from build123d import *

# Parameters (mm, degrees)
BOSS_EXTRUDE1_DEPTH = 20
SKETCH2_R           = 3.15
CUT_EXTRUDE2_DEPTH  = 11
SKETCH3_R           = 4.25
CUT_EXTRUDE3_DEPTH  = 4
BOSS_EXTRUDE2_DEPTH = 5


with BuildPart() as part:
    # Sketch1 → Boss-Extrude1 (new body)
    with BuildSketch(Plane(origin=(0, 0, 0), x_dir=(1, 0, 0), z_dir=(0, 1, 0))):
        Polygon((0, 0), (0, 43), (43, 43), (43, 0), (68, 0), (68, 10), (53, 10), (53, 53), (-10, 53), (-10, 10), (-25, 10), (-25, 0), align=None)
    extrude(amount=BOSS_EXTRUDE1_DEPTH)

    # Sketch2 → Cut-Extrude2 (cut, through all)
    with BuildSketch(Plane(origin=(0, 0, -10), x_dir=(-1, 0, 0), z_dir=(0, 0, -1))):
        with Locations((-60.5, 10)):
            Circle(SKETCH2_R)
        with Locations((17.5, 10)):
            Circle(SKETCH2_R)
    extrude(amount=-CUT_EXTRUDE2_DEPTH, mode=Mode.SUBTRACT)

    # Sketch3 → Cut-Extrude3 (cut)
    with BuildSketch(Plane(origin=(0, 0, -10), x_dir=(-1, 0, 0), z_dir=(0, 0, -1))):
        with Locations((17.5, 10)):
            Circle(SKETCH3_R)
        with Locations((-60.5, 10)):
            Circle(SKETCH3_R)
    extrude(amount=-CUT_EXTRUDE3_DEPTH, mode=Mode.SUBTRACT)

    # Sketch4 → Boss-Extrude2 (add)
    with BuildSketch(Plane.XZ):
        Polygon((-25, 5), (0, 5), (0, -43), (43, -43), (43, 5), (68, 5), (68, -10), (53, -10), (53, -53), (-10, -53), (-10, -10), (-25, -10), align=None)
    extrude(amount=BOSS_EXTRUDE2_DEPTH)


solid = part.part
Check sheet for the modelled part. Datum: model origin and axes. Units: mm. A direction names the side the tool comes from. Coordinates: 2 decimals unless noted, no trailing zeros. Loops run counter-clockwise (first coordinate to the right, second up) from the corner with the lowest first, then second, coordinate; pieces in that order, holes last. Notation, with made-up numbers: (41.25, -12) -> (92.25, -12) arc R28 ccw to (92.25, 21) -> close; hole circle Ø5 at (-18, 19.5). An arc over 180 degrees is marked (long way). Answer in a Markdown table with one row per item.
1. Sectioned sample at A-A, the plane x = 60.5. Record the boundary of the cut face in (y, z), then the cut area to 3 significant figures.
Check values:
| item | result |
|---|---|
| outline | (-5, -10) -> (5.75, -10) -> (5.75, -6) -> (6.85, -6) -> (6.85, 0) -> (0, 0) -> (0, 5) -> (-5, 5) -> close; (13.15, -6) -> (14.25, -6) -> (14.25, -10) -> (20, -10) -> (20, 0) -> (13.15, 0) -> close |
| area | 203 mm2 |
2. Sectioned sample at B-B, the plane z = -30. Record the boundary of the cut face in (x, y), then the cut area to 3 significant figures.
Check values:
| item | result |
|---|---|
| outline | (-10, -5) -> (0, -5) -> (0, 20) -> (-10, 20) -> close; (43, -5) -> (53, -5) -> (53, 20) -> (43, 20) -> close |
| area | 500 mm2 |
3. Go/stop test with flat-tipped pins: pin 1 (4 mm diameter, centred on x = 52.5, z = 2.5, fed in from +Y); pin 2 (7.5 mm diameter, centred on x = 17.5, y = 8.5, fed in from +Z); pin 3 (7.5 mm diameter, centred on x = -14.5, y = 6.5, fed in from -Z). Record where each tip stops, or that it passes through.
Check values:
| item | result |
|---|---|
| pin 1 | stops at y = 0 |
| pin 2 | stops at z = -43 |
| pin 3 | stops at z = -10 |
4. Release check for a two-part mould opening along Y. For faces 5 (the face through (55, 10, 0)), 6 (the face through (56, 0, 3)), 7 (the face through (-14.13, 7.41, -8.03)) record: released by +Y, released by -Y, zero draft, split by the parting line, or undercut.
Check values:
| item | result |
|---|---|
| face 5 | zero draft |
| face 6 | released by +Y |
| face 7 | undercut |
5. Sectioned sample at C-C, the plane y = 10. Record the boundary of the cut face in (x, z), then the cut area to 3 significant figures.
Check values:
| item | result |
|---|---|
| outline | (-25, -10) -> (-21.75, -10) -> (-21.75, -6) -> (-20.65, -6) -> (-20.65, 0) -> (-25, 0) -> close; (-14.35, -6) -> (-13.25, -6) -> (-13.25, -10) -> (-10, -10) -> (-10, -53) -> (53, -53) -> (53, -10) -> (56.25, -10) -> (56.25, -6) -> (57.35, -6) -> (57.35, 0) -> (43, 0) -> (43, -43) -> (0, -43) -> (0, 0) -> (-14.35, 0) -> close; (63.65, -6) -> (64.75, -6) -> (64.75, -10) -> (68, -10) -> (68, 0) -> (63.65, 0) -> close |
| area | 1,650 mm2 |
6. Sectioned sample at D-D, the plane z = 1. Record the boundary of the cut face in (x, y).
Check values:
| item | result |
|---|---|
| outline | (-25, -5) -> (0, -5) -> (0, 0) -> (-25, 0) -> close; (43, -5) -> (68, -5) -> (68, 0) -> (43, 0) -> close |
7. Material ranges on line 1 along X through (y, z) = (9, -30.5); line 2 along X through (y, z) = (1.5, -1.5); line 3 along Y through (x, z) = (60.5, -8.8), recorded low to high. Write a range as [from, to].
Check values:
| item | result |
|---|---|
| line 1 | x = [-10, 0], [43, 53] |
| line 2 | x = [-25, 0], [43, 68] |
| line 3 | y = [-5, 5.75], [14.25, 20] |
8. Access from +Z, -Z, +X, -X, +Y, -Y to the whole of each face (thin tool, end or side, straight path). Record for faces 1 (the face through (56.574, 8.372, -8.028)), 2 (the face through (-13, 10, 0)), 3 (the face through (21, 8, -43)), 4 (the face through (-17, 5, -10)).
Check values:
| item | result |
|---|---|
| face 1 | -Z |
| face 2 | +Z, +X, -X, +Y |
| face 3 | +Z, +Y, -Y |
| face 4 | -Z, -X, +Y, -Y |
